Work out the finished part from the listing and answer in its coordinate system (mm). Give positions to 0.01 mm unless a question says otherwise; leave off trailing zeros. Order: outer loops, then holes, each group sorted by start corner. A loop starts at its lowest first (then second) coordinate and runs counter-clockwise, first axis right, second up. Notation, with made-up numbers: (38, 38) - (67, 38) arc R20 ccw to (67, 72) - close; hole circle Ø4 at (11, 11.5). An arc over 180 degrees is marked (long way). Return JSON: item names as keys, results as strings. Group by question number.
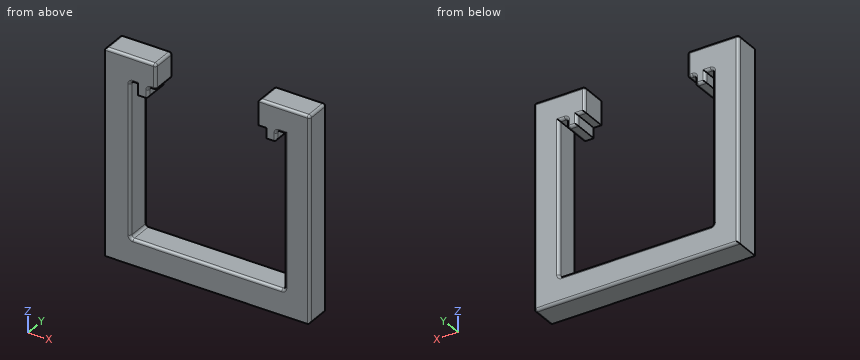
from build123d import *

# Parameters (mm, degrees)
SKETCH1_W           = 2
SKETCH1_H           = 2
BOSS_EXTRUDE1_DEPTH = 5
FILLET1_R           = 0.5


with BuildPart() as part:
    # Sketch1 → Boss-Extrude1 (new body)
    with BuildSketch(Plane(origin=(0, 0, 0), x_dir=(1, 0, 0), z_dir=(0, 1, 0))):
        Polygon((-53.419958922, -370.98752745), (-61.112267161, -370.98752745), (-61.112267161, -380.152018312), (-61.112267161, -410.98752745), (-56.112267161, -410.98752745), (-56.112267161, -405.98752745), (-56.112267161, -375.98752745), (-26.112267161, -375.98752745), (-26.112267161, -405.98752745), (-26.112267161, -410.98752745), (-21.112267161, -410.98752745), (-21.112267161, -380.152018312), (-21.112267161, -370.98752745), align=None)
        Polygon((-56.112267161, -405.98752745), (-56.112267161, -410.98752745), (-51.112267161, -410.98752745), (-51.112267161, -405.98752745), (-52.612267161, -405.98752745), (-54.612267161, -405.98752745), align=None)
        Polygon((-31.112267161, -410.98752745), (-26.112267161, -410.98752745), (-26.112267161, -405.98752745), (-27.612267161, -405.98752745), (-29.612267161, -405.98752745), (-31.112267161, -405.98752745), align=None)
        with Locations((-53.612267161, -404.98752745)):
            Rectangle(SKETCH1_W, SKETCH1_H)
        with Locations((-28.612267161, -404.98752745)):
            Rectangle(SKETCH1_W, SKETCH1_H)
    extrude(amount=BOSS_EXTRUDE1_DEPTH)

    # Fillet1
    fillet1_edges = [part.edges().sort_by_distance(p)[0] for p in [
        (-27.612267161, 5, 404.98752745),
        (-28.612267161, 5, 403.98752745),
        (-41.112267161, 0, 375.98752745),
        (-56.112267161, 0, 390.98752745),
        (-55.362267161, 0, 405.98752745),
        (-29.612267161, 5, 404.98752745),
        (-52.612267161, 0, 404.98752745),
        (-51.862267161, 0, 405.98752745),
        (-51.112267161, 0, 408.48752745),
        (-56.112267161, 0, 410.98752745),
        (-30.362267161, 5, 405.98752745),
        (-21.112267161, 0, 390.98752745),
        (-26.112267161, 0, 410.98752745),
        (-31.112267161, 5, 408.48752745),
        (-27.612267161, 0, 404.98752745),
        (-26.862267161, 0, 405.98752745),
        (-26.112267161, 0, 390.98752745),
        (-26.112267161, 5, 410.98752745),
        (-26.112267161, 2.5, 375.98752745),
        (-56.112267161, 2.5, 375.98752745),
        (-56.112267161, 2.5, 405.98752745),
        (-52.612267161, 2.5, 403.98752745),
        (-52.612267161, 2.5, 405.98752745),
        (-51.112267161, 2.5, 405.98752745),
        (-51.112267161, 2.5, 410.98752745),
        (-61.112267161, 2.5, 410.98752745),
        (-21.112267161, 2.5, 370.98752745),
        (-21.112267161, 2.5, 410.98752745),
        (-31.112267161, 2.5, 410.98752745),
        (-27.612267161, 2.5, 403.98752745),
        (-27.612267161, 2.5, 405.98752745),
        (-26.112267161, 5, 390.98752745),
        (-21.112267161, 5, 390.98752745),
        (-41.112267161, 5, 370.98752745),
        (-61.112267161, 5, 390.98752745),
        (-56.112267161, 5, 410.98752745),
        (-51.112267161, 5, 408.48752745),
        (-51.862267161, 5, 405.98752745),
        (-52.612267161, 5, 404.98752745),
        (-53.612267161, 5, 403.98752745),
        (-54.612267161, 5, 404.98752745),
        (-55.362267161, 5, 405.98752745),
        (-56.112267161, 5, 390.98752745),
        (-26.862267161, 5, 405.98752745),
        (-41.112267161, 5, 375.98752745),
    ]]
    fillet(fillet1_edges, radius=FILLET1_R)


solid = part.part
1. Consider probe 1 along X at (y, z) = (4.1, 405); probe 2 along X at (y, z) = (0.4, 383.5); probe 3 along Z at (x, y) = (-30, 1.4). Determine where each line is inside the solid, lowest interval first. Write a range as from..to.
2. The part is cut by section A-A (z = 389.5). Give the vertices of the cut face in (x, y).
3. Each of these flat-tipped pins is pushed along its axis until it touches: pin 1 (3 mm diameter, centred on x = -39.5, y = 3.5, fed in from +Z); pin 2 (8 mm diameter, centred on x = -54, z = 402.5, fed in from +Y). Where does it stop, or does it pass through?
4. The part is cut by section C-C (x = -39). Give the vertices of the cut face in (y, z).
Answers:
{
 "1": {"probe 1": "x = -61.11..-56.11, -54.61..-52.61, -29.61..-27.61, -26.11..-21.11", "probe 2": "x = -61.11..-56.12, -26.1..-21.12", "probe 3": "z = 370.99..375.99, 405.99..410.99"},
 "2": {"outline": "(-61.11, 0) - (-56.61, 0) arc R0.5 ccw to (-56.11, 0.5) - (-56.11, 4.5) arc R0.5 ccw to (-56.61, 5) - (-60.61, 5) arc R0.5 ccw to (-61.11, 4.5) - close; (-26.11, 0.5) arc R0.5 ccw to (-25.61, 0) - (-21.61, 0) arc R0.5 ccw to (-21.11, 0.5) - (-21.11, 4.5) arc R0.5 ccw to (-21.61, 5) - (-25.61, 5) arc R0.5 ccw to (-26.11, 4.5) - close"},
 "3": {"pin 1": "stops at z = 375.99", "pin 2": "stops at y = 5"},
 "4": {"outline": "(0, 370.99) - (4.5, 370.99) arc R0.5 ccw to (5, 371.49) - (5, 375.49) arc R0.5 ccw to (4.5, 375.99) - (0.5, 375.99) arc R0.5 ccw to (0, 375.49) - close"}
}
